Read the model definition and answer for the solid it produces. Units are mm, in the model's axes. A direction names the side the tool comes from. Give positions to 0.01 mm unless a question says otherwise; leave off trailing zeros. Order: outer loops, then holes, each group sorted by start corner. A loop starts at its lowest first (then second) coordinate and runs counter-clockwise, first axis right, second up. Notation, with made-up numbers: M -21.5,39 L 22.5,39 A26 cw 22.5,74 Z; hole C 38,17 d7. An arc over 180 degrees is marked long. Write item = value, one per line. Start each with the question number.
Autodesk Inventor part; units mm, degrees
ref_plane "YZ Plane" through (0, 0, 0) normal (1, 0, 0) x (0, 1, 0)
ref_plane "XZ Plane" through (0, 0, 0) normal (0, 1, 0) x (-1, 0, 0)
ref_plane "XY Plane" through (0, 0, 0) normal (0, 0, 1) x (1, 0, 0)
sketch "Sketch1" plane through (0, 0, 0) normal (0, 0, 1) x (1, 0, 0)
  line L0 (0, 0) -> (39.7, 0)
  circle A0 centre (43.66, 15) radius 1.5
  circle A1 centre (43.66, 4.8) radius 1.5
  circle A2 centre (-3.96, 15) radius 1.5
  circle A3 centre (-3.96, 4.8) radius 1.5
  line L1 (46.2, 9.9) -> (46.2, 10.4)
  line L2 (46.2, 10.4) -> (39.7, 10.4)
  line L3 (46.2, 9.9) -> (46.2, 9.4)
  line L4 (46.2, 9.4) -> (39.7, 9.4)
  line L5 (39.7, 0) -> (39.7, 9.4)
  line L6 (39.7, 10.4) -> (39.7, 18.8)
  line L7 (-6.5, 9.9) -> (-6.5, 10.4)
  line L8 (-6.5, 10.4) -> (0, 10.4)
  line L9 (-6.5, 9.4) -> (0, 9.4)
  line L10 (-6.5, 9.9) -> (-6.5, 9.4)
  line L11 (0, 9.4) -> (0, 0)
  line L12 (29.8, -3.5) -> (31.05, -3.5)
  line L13 (31.05, -23.3) -> (28.55, -23.3)
  line L14 (28.55, -23.3) -> (28.55, -3.5)
  line L15 (28.55, -3.5) -> (29.8, -3.5)
  line L16 (29.8, -23.3) -> (29.8, -28.3)
  circle A4 centre (29.8, -28.3) radius 1.5
  line L17 (31.05, -23.3) -> (31.05, -13.9)
  line L18 (31.05, -13.9) -> (33.55, -13.9)
  line L19 (33.55, -13.9) -> (33.55, -12.9)
  line L20 (33.55, -12.9) -> (31.05, -12.9)
  line L21 (31.05, -12.9) -> (31.05, -3.5)
  line L22 (36.55, -14.9) -> (36.55, -28.3)
  line L23 (-10, 0) -> (-10, -3)
  line L24 (36.55, -13) -> (36.55, -14.9)
  line L25 (41.55, -8) -> (44.7, -8)
  line L26 (49.7, -3) -> (49.7, 0)
  arc A5 (24.55, -28.3) -> (36.55, -28.3) centre (30.55, -28.3) ccw
  arc A6 (44.7, -8) -> (49.7, -3) centre (44.7, -3) ccw
  arc A7 (-10, -3) -> (-5, -8) centre (-5, -3) ccw
  arc A8 (41.55, -8) -> (36.55, -13) centre (41.55, -13) ccw
  line L27 (24.55, -28.6619) -> (24.55, -28.3)
  line L28 (-3.2198, -8) -> (-5, -8)
  line L29 (1.9251, -9.4251) -> (19.695, -20.087)
  arc A9 (1.9251, -9.4251) -> (-3.2198, -8) centre (-3.2198, -18) ccw
  arc A10 (24.55, -28.6619) -> (19.695, -20.087) centre (14.55, -28.6619) ccw
  line L30 (-2, 20.8) -> (-8, 20.8)
  line L31 (-10, 18.8) -> (-10, 0)
  line L32 (41.7, 20.8) -> (47.7, 20.8)
  line L33 (49.7, 18.8) -> (49.7, 0)
  arc A11 (0, 18.8) -> (-2, 20.8) centre (-2, 18.8) ccw
  arc A12 (-8, 20.8) -> (-10, 18.8) centre (-8, 18.8) ccw
  arc A13 (41.7, 20.8) -> (39.7, 18.8) centre (41.7, 18.8) ccw
  arc A14 (49.7, 18.8) -> (47.7, 20.8) centre (47.7, 18.8) ccw
  line L34 (0, 18.8) -> (0, 10.4)
  point P0 (0, 20.8)
  point P1 (-10, 20.8)
  dimension "d13" = 1.25
  dimension "d15" = 2.5
  dimension "d16" = 19.8
  dimension "d17" = 5
  dimension "d25" = 9.4
  dimension "d26" = 2.5
  dimension "d27" = 1
  dimension "d28" = 1
  dimension "d29" = 1
  dimension "d30" = 6.5
  dimension "d48" = 5
  dimension "d54" = 10
  dimension "d57" = 10
  dimension "d58" = 2
extrude "Extrusion1" add sketch "Sketch1" along normal blind 5
properties part number "braket atas 2"
1) Find section B-B on x = 43.66. Determine the outline of the cut face in (y, z).
2) For a pull along Y with two mould halves and no side action, classify faces 1 (the face through (31.05, -8, 2)), 2 (the face through (-4, -8, 2)), 3 (the face through (0, 15, 2)) as pulls with the +Y half, pulls with the -Y half, needs draft (parallel to the pull), parting line crosses it, or undercut.
3) For faces 4 (the face through (39.7, 15, 2)), 5 (the face through (30, -3.5, 2)), 6 (the face through (10.686, -14.681, 2.465)), determine the directions among +Z, -Z, +X, -X, +Y, -Y from which every point of the face is accessible in a straight line to the end or side of a thin tool.
4) Find section D-D on x = -1. Determine the outline of the cut face in (y, z).
5) Find the intervals of material crossed by probe 1 along Y at (x, z) = (43.66, 3.35); probe 2 along X at (y, z) = (6, 3.95); probe 3 along Y at (x, z) = (29.8, 2.5), in increasing order. Write a range as [from, to].
6) Each of these flat-tipped pins is pushed along its axis until it touches: P1, Ø2.5, axis at x = 43.5, z = 2.5, coming from the -Y side; P2, Ø2.5, axis at x = 32.5, z = 2, coming from the +Y side; P3, Ø3, axis at y = -24, z = 2, coming from the +X side; P4, Ø1.8, axis at x = 43.66, y = 4.8, coming from the -Z side. Where does it stop, or does it pass through?
7) Find section C-C on y = -4.5. Determine the outline of the cut face in (x, z), plus the area to 3 significant figures.
8) Find section A-A on y = 15. Determine the outline of the cut face in (x, z).
Numbers:
q1.outline = M -8,0 L 3.3,0 L 3.3,5 L -8,5 Z; M 6.3,0 L 9.4,0 L 9.4,5 L 6.3,5 Z; M 10.4,0 L 13.5,0 L 13.5,5 L 10.4,5 Z; M 16.5,0 L 20.8,0 L 20.8,5 L 16.5,5 Z
q2.face_1 = undercut
q2.face_2 = pulls with the -Y half
q2.face_3 = needs draft
q3.face_4 = +Z, -Z, +Y
q3.face_5 = +Z, -Z
q3.face_6 = +Z, -Z, -X, -Y
q4.outline = M -8.25,0 L 9.4,0 L 9.4,5 L -8.25,5 Z; M 10.4,0 L 20.53,0 L 20.53,5 L 10.4,5 Z
q5.probe_1 = [-8, 3.3], [6.3, 9.4], [10.4, 13.5], [16.5, 20.8]
q5.probe_2 = [-10, -4.86], [-3.06, 0], [39.7, 42.76], [44.56, 49.7]
q5.probe_3 = [-34.25, -29.8], [-26.8, -23.3], [-3.5, 0]
q6.P1 = -8
q6.P2 = 0
q6.P3 = 36.55
q6.P4 = through
q7.outline = M -9.77,0 L 28.55,0 L 28.55,5 L -9.77,5 Z; M 31.05,0 L 49.47,0 L 49.47,5 L 31.05,5 Z
q7.area = 284 mm2
q8.outline = M -10,0 L -5.46,0 L -5.46,5 L -10,5 Z; M -2.46,0 L 0,0 L 0,5 L -2.46,5 Z; M 39.7,0 L 42.16,0 L 42.16,5 L 39.7,5 Z; M 45.16,0 L 49.7,0 L 49.7,5 L 45.16,5 Z
